from build123d import *

# Parameters (mm, degrees)
F0_R         = 4
F1_DEPTH     = 7
F3_DEPTH     = 25
F4_T1_DEPTH  = 26
F4_T3_DEPTH  = 1
F4_T5_DEPTH  = 10.285841494
F4_T7_DEPTH  = 12.4424386412
F4_T9_DEPTH  = 11.029084367
F4_T12_ANGLE = 90
F4_T14_ANGLE = 90
F4_T16_ANGLE = 90
F4_T18_ANGLE = 90
F4_T24_ANGLE = 90
F4_T26_ANGLE = 90
F4_T30_ANGLE = 90
F4_T32_ANGLE = 90


# Not quite as in the source:
# - a fillet or chamfer that OpenCascade refuses, or shapes differently, is made with other operations: its cross-section is extruded or revolved along the edge and cut away or added


with BuildPart() as f1:
    # F0 (on Top) → F1 (new body)
    with BuildSketch(Plane.XY):
        with BuildLine():
            Line((25.5, 5.5), (-0.5, 5.5))
            ThreePointArc((-0.5, 5.5), (-4.0355339059, 4.0355339059), (-5.5, 0.5))
            Line((-5.5, 0.5), (-5.5, -0.5))
            ThreePointArc((-5.5, -0.5), (-4.0355339059, -4.0355339059), (-0.5, -5.5))
            Line((-0.5, -5.5), (25.5, -5.5))
            ThreePointArc((25.5, -5.5), (29.0355339059, -4.0355339059), (30.5, -0.5))
            Line((30.5, -0.5), (30.5, 0.5))
            ThreePointArc((30.5, 0.5), (29.0355339059, 4.0355339059), (25.5, 5.5))
        make_face()
        Circle(F0_R, mode=Mode.SUBTRACT)
        with Locations((25, 0)):
            Circle(F0_R, mode=Mode.SUBTRACT)
    extrude(amount=F1_DEPTH)

    # F2 (on face) → F3 (cut)
    with BuildSketch(Plane.XZ.offset(5.5)):
        with BuildLine():
            Line((15.756757127, 7), (8.5, 7))
            ThreePointArc((8.5, 7), (12.1283785635, 4.963), (15.756757127, 7))
        make_face()
    extrude(amount=-F3_DEPTH, mode=Mode.SUBTRACT)

    # F4: chamfer of 0.5 on 24 edges, made by hand

    # F4_s2 → F4_t1 (cut)
    with BuildSketch(Plane.YZ.offset(-0.5)):
        Polygon((-5, 0), (-5.5, 0.5), (-5.5, 0), align=None)
        Polygon((5, 0), (5.5, 0.5), (5.5, 0), align=None)
    extrude(amount=F4_T1_DEPTH, mode=Mode.SUBTRACT)

    # F4_s4 → F4_t3 (cut)
    with BuildSketch(Plane.XZ.offset(-0.5)):
        Polygon((30.5, 0.5), (30, 0), (30.5, 0), align=None)
        Polygon((-5, 0), (-5.5, 0.5), (-5.5, 0), align=None)
        Polygon((-5.5, 6.5), (-5, 7), (-5.5, 7), align=None)
        Polygon((30.5, 6.5), (30, 7), (30.5, 7), align=None)
    extrude(amount=F4_T3_DEPTH, mode=Mode.SUBTRACT)

    # F4_s6 → F4_t5 (cut)
    with BuildSketch(Plane.YZ.offset(-0.5)):
        Polygon((-5.5, 6.5), (-5, 7), (-5.5, 7), align=None)
        Polygon((5.5, 6.5), (5, 7), (5.5, 7), align=None)
    extrude(amount=F4_T5_DEPTH, mode=Mode.SUBTRACT)

    # F4_s8 → F4_t7 (cut)
    with BuildSketch(Plane.XZ.offset(-6.2212193206)):
        with BuildLine():
            Line((8.6398076479, 6.7855789474), (8.2293875402, 7))
            Line((8.2293875402, 7), (8.5, 7))
            ThreePointArc((8.5, 7), (8.5730669131, 6.8844255286), (8.6398076479, 6.7855789474))
        make_face()
        with BuildLine():
            Line((16.0273695868, 7), (15.6169494791, 6.7855789474))
            ThreePointArc((15.6169494791, 6.7855789474), (15.6836902138, 6.8844255286), (15.756757127, 7))
            Line((15.756757127, 7), (16.0273695868, 7))
        make_face()
    extrude(amount=F4_T7_DEPTH, mode=Mode.SUBTRACT)

    # F4_s10 → F4_t9 (cut)
    with BuildSketch(Plane.YZ.offset(14.470915633)):
        Polygon((-5, 7), (-5.5, 6.5), (-5.5, 7), align=None)
        Polygon((5, 7), (5.5, 6.5), (5.5, 7), align=None)
    extrude(amount=F4_T9_DEPTH, mode=Mode.SUBTRACT)

    # F4_s11 → F4_t12 (revolve, cut)
    with BuildSketch(Plane.XZ.offset(-0.5)):
        Polygon((30.5, 0.5), (30, 0), (30.5, 0), align=None)
    revolve(axis=Axis((25.5, 0.5, 0), (0, 0, 1)), revolution_arc=F4_T12_ANGLE, mode=Mode.SUBTRACT)

    # F4_s13 → F4_t14 (revolve, cut)
    with BuildSketch(Plane.YZ.offset(-0.5)):
        Polygon((5, 0), (5.5, 0.5), (5.5, 0), align=None)
    revolve(axis=Axis((-0.5, 0.5, 0), (0, 0, 1)), revolution_arc=F4_T14_ANGLE, mode=Mode.SUBTRACT)

    # F4_s15 → F4_t16 (revolve, cut)
    with BuildSketch(Plane.XZ.offset(0.5)):
        Polygon((-5, 0), (-5.5, 0.5), (-5.5, 0), align=None)
    revolve(axis=Axis((-0.5, -0.5, 0), (0, 0, 1)), revolution_arc=F4_T16_ANGLE, mode=Mode.SUBTRACT)

    # F4_s17 → F4_t18 (revolve, cut)
    with BuildSketch(Plane.YZ.offset(25.5)):
        Polygon((-5.5, 0.5), (-5, 0), (-5.5, 0), align=None)
    revolve(axis=Axis((25.5, -0.5, 0), (0, 0, 1)), revolution_arc=F4_T18_ANGLE, mode=Mode.SUBTRACT)

    # F4_s19 → F4_t20 (revolve, cut)
    with BuildSketch(Plane.XZ):
        Polygon((4.5, 0), (4, 0.5), (4, 0), align=None)
    revolve(axis=Axis((0, 0, 0), (0, 0, 1)), mode=Mode.SUBTRACT)

    # F4_s21 → F4_t22 (revolve, cut)
    with BuildSketch(Plane.XZ):
        Polygon((29.5, 0), (29, 0.5), (29, 0), align=None)
    revolve(axis=Axis((25, 0, 0), (0, 0, 1)), mode=Mode.SUBTRACT)

    # F4_s23 → F4_t24 (revolve, cut)
    with BuildSketch(Plane.XZ.offset(0.5)):
        Polygon((-5.5, 6.5), (-5, 7), (-5.5, 7), align=None)
    revolve(axis=Axis((-0.5, -0.5, 7), (0, 0, 1)), revolution_arc=F4_T24_ANGLE, mode=Mode.SUBTRACT)

    # F4_s25 → F4_t26 (revolve, cut)
    with BuildSketch(Plane.YZ.offset(-0.5)):
        Polygon((5.5, 6.5), (5, 7), (5.5, 7), align=None)
    revolve(axis=Axis((-0.5, 0.5, 7), (0, 0, 1)), revolution_arc=F4_T26_ANGLE, mode=Mode.SUBTRACT)

    # F4_s27 → F4_t28 (revolve, cut)
    with BuildSketch(Plane.XZ):
        Polygon((4, 6.5), (4.5, 7), (4, 7), align=None)
    revolve(axis=Axis((0, 0, 7), (0, 0, 1)), mode=Mode.SUBTRACT)

    # F4_s29 → F4_t30 (revolve, cut)
    with BuildSketch(Plane.YZ.offset(25.5)):
        Polygon((-5.5, 6.5), (-5, 7), (-5.5, 7), align=None)
    revolve(axis=Axis((25.5, -0.5, 7), (0, 0, 1)), revolution_arc=F4_T30_ANGLE, mode=Mode.SUBTRACT)

    # F4_s31 → F4_t32 (revolve, cut)
    with BuildSketch(Plane.XZ.offset(-0.5)):
        Polygon((30.5, 6.5), (30, 7), (30.5, 7), align=None)
    revolve(axis=Axis((25.5, 0.5, 7), (0, 0, 1)), revolution_arc=F4_T32_ANGLE, mode=Mode.SUBTRACT)

    # F4_s33 → F4_t34 (revolve, cut)
    with BuildSketch(Plane.XZ):
        Polygon((29.5, 7), (29, 6.5), (29, 7), align=None)
    revolve(axis=Axis((25, 0, 7), (0, 0, 1)), mode=Mode.SUBTRACT)


solid = f1.part
The listing builds one solid part. Answer for the finished solid, in the listing's coordinates (mm). Coordinates: 2 decimals unless noted, no trailing zeros. Write each loop counter-clockwise with the first axis right and the second up, starting at its lowest first coordinate (ties: lowest second). Pieces come first, ordered by that corner, then holes. Notation, with made-up numbers: (20.25, 73) - (36.25, 73) arc R28 cw to (36.25, 103) - close; hole circle Ø8 at (44.5, 28). An arc over 180 degrees is marked (long way). Put each result on its own line as item: value.
1. A flat-ended cylindrical pin translates along its axis: pin 1 Ø2 at (x, y) = (0, 2) entering from +Z. Find the tip coordinate at first contact, or state that the pin passes through.
Answer sheet:
pin 1: passes through
2. Determine the mould class of faces 1 (the face through (-3.819, -3.746, 0.142)), 2 (the face through (13, 5.5, 3)), 3 (the face through (-0.867, -3.905, 3.458)) for opening direction X: pulls with the +X half, pulls with the -X half, needs draft (parallel to the pull), parting line crosses it, or undercut.
Answer sheet:
face 1: pulls with the -X half
face 2: needs draft
face 3: undercut
3. The part is cut by section B-B on x = 0. Give the vertices of the cut face in (y, z).
Answer sheet:
outline: (-5.5, 0.5) - (-5, 0) - (-4.5, 0) - (-4, 0.5) - (-4, 6.5) - (-4.5, 7) - (-5, 7) - (-5.5, 6.5) - close; (4, 0.5) - (4.5, 0) - (5, 0) - (5.5, 0.5) - (5.5, 6.5) - (5, 7) - (4.5, 7) - (4, 6.5) - close
4. The part is cut by section D-D on y = 2.75. State how many separate pieces and enclosed holes the cut face has, plus the area to 3 significant figures.
Answer sheet:
separate pieces: 3
enclosed holes: 0
area: 151 mm^2
5. The part is cut by section A-A on y = 0. Give the vertices of the cut face in (x, z).
Answer sheet:
outline: (-5.5, 0.5) - (-5, 0) - (-4.5, 0) - (-4, 0.5) - (-4, 6.5) - (-4.5, 7) - (-5, 7) - (-5.5, 6.5) - close; (4, 0.5) - (4.5, 0) - (20.5, 0) - (21, 0.5) - (21, 6.5) - (20.5, 7) - (16.03, 7) - (15.62, 6.79) arc R4.25 cw to (8.64, 6.79) - (8.23, 7) - (4.5, 7) - (4, 6.5) - close; (29, 0.5) - (29.5, 0) - (30, 0) - (30.5, 0.5) - (30.5, 6.5) - (30, 7) - (29.5, 7) - (29, 6.5) - close
6. The part is cut by section C-C on z = 2.5. Give the vertices of the cut face in (x, y).
Answer sheet:
outline: (-5.5, -0.5) arc R5 ccw to (-0.5, -5.5) - (25.5, -5.5) arc R5 ccw to (30.5, -0.5) - (30.5, 0.5) arc R5 ccw to (25.5, 5.5) - (-0.5, 5.5) arc R5 ccw to (-5.5, 0.5) - close; hole circle Ø8 at (0, 0); hole circle Ø8 at (25, 0)
7. Find the intervals of material crossed by line 1 along Y through (x, z) = (0, 5.1); line 2 along X through (y, z) = (-3.5, 4.25); line 3 along X through (y, z) = (-3, 0.75), in increasing order. Write a range as from..to.
Answer sheet:
line 1: y = -5.5..-4, 4..5.5
line 2: x = -4.5..-1.94, 1.94..23.06, 26.94..29.5
line 3: x = -4.83..-2.65, 2.65..22.35, 27.65..29.83
